```python
from build123d import *

# Parameters (mm, degrees)
F1_DEPTH = 44
F0_W     = 14
F0_H     = 12
F2_DEPTH = 25


with BuildPart() as f1:
    # F0 (on Front) → F1 (new body)
    with BuildSketch(Plane.XZ):
        Polygon((51.345316, 25), (-18.654684, 25), (-18.654684, 13), (-18.654684, 0), (1.345316, -40), (31.345316, -40), (51.345316, 0), (51.345316, 13), align=None)
    extrude(amount=F1_DEPTH)

    # F0 (on Front) → F2 (join)
    with BuildSketch(Plane.XZ):
        with Locations((-25.654684, 19)):
            Rectangle(F0_W, F0_H)
        with Locations((58.345316, 19)):
            Rectangle(F0_W, F0_H)
    extrude(amount=F2_DEPTH)


solid = f1.part
```
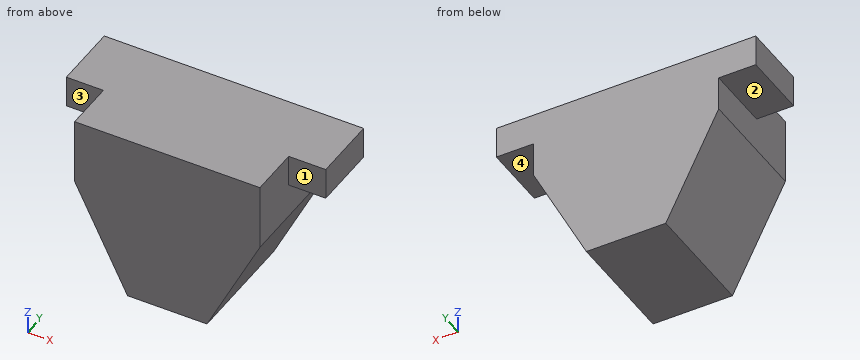
The model under review builds one solid part; all positions refer to its coordinate system, in mm. Face numbers are marked on the shaded views. A direction names the side the tool comes from. Give positions to 0.01 mm unless a question says otherwise; leave off trailing zeros. Write each loop counter-clockwise with the first axis right and the second up, starting at its lowest first coordinate (ties: lowest second). Pieces come first, ordered by that corner, then holes. Notation, with made-up numbers: M 81,13 L 111,13 A15 ccw 111,17 Z; hole C 32,62 d11. An arc over 180 degrees is marked long. Write item = value, one per line. Start each with the question number.
Q1. We need section B-B (x = -20). State the section outline as (y, z) points, plus the area to 3 significant figures.
Q2. We need section A-A (y = -19.5). State the section outline as (x, z) points.
Q3. We need section D-D (y = -27.5). State the section outline as (x, z) points.
Q4. Machinability: for the marked faces 1, 2, 3 and 4, which of the approach directions +Z, -Z, +X, -X, +Y, -Y give a long, thin tool a straight path to every point of the face, cutting with its end or side? Answer none if there is none.
Q5. For line 1 (X direction, y = -42, z = 21); line 2 (Z direction, x = 52.5, y = -15.5); line 3 (Z direction, x = -18.5, y = -31), list the stretches that pass through material, from the lowest coordinate up.
Q6. Clearance check with flat-ended pins moving along their axes: pin 1 (3.5 mm diameter, centred on x = 60.5, z = 21, fed in from -Y); pin 2 (7 mm diameter, centred on x = -24, y = -8.5, fed in from -Z); pin 3 (8 mm diameter, centred on y = -25, z = -9, fed in from -X). State where each tip first meets the part, or that it passes through.
Q7. We need section C-C (z = 10). State the section outline as (x, y) points, plus the area to 3 significant figures.
Result set:
q1.outline = M -25,13 L 0,13 L 0,25 L -25,25 Z
q1.area = 300 mm2
q2.outline = M -32.65,13 L -18.65,13 L -18.65,0 L 1.35,-40 L 31.35,-40 L 51.35,0 L 51.35,13 L 65.35,13 L 65.35,25 L -32.65,25 Z
q3.outline = M -18.65,0 L 1.35,-40 L 31.35,-40 L 51.35,0 L 51.35,25 L -18.65,25 Z
q4.face_1 = +Z, -Z, +X, -Y
q4.face_2 = -Z, -X, +Y, -Y
q4.face_3 = +Z, -Z, -X, -Y
q4.face_4 = -Z, +X, +Y, -Y
q5.line_1 = -18.65 to 51.35
q5.line_2 = 13 to 25
q5.line_3 = -0.31 to 25
q6.pin_1 = -25
q6.pin_2 = 13
q6.pin_3 = -16.15
q7.outline = M -18.65,-44 L 51.35,-44 L 51.35,0 L -18.65,0 Z
q7.area = 3,080 mm2
